Autodesk Inventor part; units mm, degrees
ref_plane "YZ Plane" through (0, 0, 0) normal (1, 0, 0) x (0, 1, 0)
ref_plane "XZ Plane" through (0, 0, 0) normal (0, 1, 0) x (-1, 0, 0)
ref_plane "XY Plane" through (0, 0, 0) normal (0, 0, 1) x (1, 0, 0)
sketch "Эскиз1" plane through (0, 0, 0) normal (0, 0, 1) x (1, 0, 0)
  arc A0 (130.1731, 0.7623) -> (123.4106, 7.5248) centre (123.4106, 0.7623) ccw
  line L0 (-123.2839, 7.5248) -> (123.4106, 7.5248)
  arc A1 (-123.2839, 7.5248) -> (-130.0464, 0.7623) centre (-123.2839, 0.7623) ccw
  line L1 (-130.0464, -1.7127) -> (-130.0464, 0.7623)
  arc A2 (-130.0464, -1.7127) -> (-123.2839, -8.4752) centre (-123.2839, -1.7127) ccw
  line L2 (123.4106, -8.4752) -> (-123.2839, -8.4752)
  arc A3 (123.4106, -8.4752) -> (130.1731, -1.7127) centre (123.4106, -1.7127) ccw
  line L3 (130.1731, 0.7623) -> (130.1731, -1.7127)
  circle A4 centre (122.1731, -0.4752) radius 1.85
  circle A5 centre (-124.1763, -0.4762) radius 1.65
  circle A6 centre (-106.5766, -0.4757) radius 2.65
  circle A7 centre (-92.1769, -0.4756) radius 1.65
  line L4 (-73.2645, 4.044) -> (-78.5234, -4.9714)
  arc A8 (-71.5369, 4.044) -> (-73.2645, 4.044) centre (-72.4007, 3.5401) ccw
  line L5 (-66.2779, -4.9714) -> (-71.5369, 4.044)
  arc A9 (-67.1417, -6.4752) -> (-66.2779, -4.9714) centre (-67.1417, -5.4752) ccw
  line L6 (-77.6596, -6.4752) -> (-67.1417, -6.4752)
  arc A10 (-78.5234, -4.9714) -> (-77.6596, -6.4752) centre (-77.6596, -5.4752) ccw
  line L7 (-57.8267, 5.5248) -> (-68.3446, 5.5248)
  arc A11 (-56.9629, 4.0209) -> (-57.8267, 5.5248) centre (-57.8267, 4.5248) ccw
  line L8 (-62.2219, -4.9945) -> (-56.9629, 4.0209)
  arc A12 (-63.9495, -4.9945) -> (-62.2219, -4.9945) centre (-63.0857, -4.4906) ccw
  line L9 (-69.2084, 4.0209) -> (-63.9495, -4.9945)
  arc A13 (-68.3446, 5.5248) -> (-69.2084, 4.0209) centre (-68.3446, 4.5248) ccw
  line L10 (-54.634, 4.044) -> (-59.893, -4.9714)
  arc A14 (-52.9065, 4.044) -> (-54.634, 4.044) centre (-53.7703, 3.5401) ccw
  line L11 (-47.6475, -4.9714) -> (-52.9065, 4.044)
  arc A15 (-48.5113, -6.4752) -> (-47.6475, -4.9714) centre (-48.5113, -5.4752) ccw
  line L12 (-59.0292, -6.4752) -> (-48.5113, -6.4752)
  arc A16 (-59.893, -4.9714) -> (-59.0292, -6.4752) centre (-59.0292, -5.4752) ccw
  line L13 (-39.1963, 5.5248) -> (-49.7142, 5.5248)
  arc A17 (-38.3325, 4.0209) -> (-39.1963, 5.5248) centre (-39.1963, 4.5248) ccw
  line L14 (-43.5915, -4.9945) -> (-38.3325, 4.0209)
  arc A18 (-45.319, -4.9945) -> (-43.5915, -4.9945) centre (-44.4553, -4.4906) ccw
  line L15 (-50.578, 4.0209) -> (-45.319, -4.9945)
  arc A19 (-49.7142, 5.5248) -> (-50.578, 4.0209) centre (-49.7142, 4.5248) ccw
  line L16 (-36.0036, 4.044) -> (-41.2626, -4.9714)
  arc A20 (-34.2761, 4.044) -> (-36.0036, 4.044) centre (-35.1399, 3.5401) ccw
  line L17 (-29.0171, -4.9714) -> (-34.2761, 4.044)
  arc A21 (-29.8809, -6.4752) -> (-29.0171, -4.9714) centre (-29.8809, -5.4752) ccw
  line L18 (-40.3988, -6.4752) -> (-29.8809, -6.4752)
  arc A22 (-41.2626, -4.9714) -> (-40.3988, -6.4752) centre (-40.3988, -5.4752) ccw
  line L19 (-20.5659, 5.5248) -> (-31.0838, 5.5248)
  arc A23 (-19.7021, 4.0209) -> (-20.5659, 5.5248) centre (-20.5659, 4.5248) ccw
  line L20 (-24.9611, -4.9945) -> (-19.7021, 4.0209)
  arc A24 (-26.6886, -4.9945) -> (-24.9611, -4.9945) centre (-25.8249, -4.4906) ccw
  line L21 (-31.9476, 4.0209) -> (-26.6886, -4.9945)
  arc A25 (-31.0838, 5.5248) -> (-31.9476, 4.0209) centre (-31.0838, 4.5248) ccw
  line L22 (-17.3732, 4.044) -> (-22.6322, -4.9714)
  arc A26 (-15.6457, 4.044) -> (-17.3732, 4.044) centre (-16.5095, 3.5401) ccw
  line L23 (-10.3867, -4.9714) -> (-15.6457, 4.044)
  arc A27 (-11.2505, -6.4752) -> (-10.3867, -4.9714) centre (-11.2505, -5.4752) ccw
  line L24 (-21.7684, -6.4752) -> (-11.2505, -6.4752)
  arc A28 (-22.6322, -4.9714) -> (-21.7684, -6.4752) centre (-21.7684, -5.4752) ccw
  line L25 (-1.9355, 5.5248) -> (-12.4534, 5.5248)
  arc A29 (-1.0717, 4.0209) -> (-1.9355, 5.5248) centre (-1.9355, 4.5248) ccw
  line L26 (-6.3307, -4.9945) -> (-1.0717, 4.0209)
  arc A30 (-8.0582, -4.9945) -> (-6.3307, -4.9945) centre (-7.1945, -4.4906) ccw
  line L27 (-13.3172, 4.0209) -> (-8.0582, -4.9945)
  arc A31 (-12.4534, 5.5248) -> (-13.3172, 4.0209) centre (-12.4534, 4.5248) ccw
  line L28 (113.0396, 4.044) -> (107.7807, -4.9714)
  arc A32 (114.7672, 4.044) -> (113.0396, 4.044) centre (113.9034, 3.5401) ccw
  line L29 (120.0261, -4.9714) -> (114.7672, 4.044)
  arc A33 (119.1624, -6.4752) -> (120.0261, -4.9714) centre (119.1624, -5.4752) ccw
  line L30 (108.6444, -6.4752) -> (119.1624, -6.4752)
  arc A34 (107.7807, -4.9714) -> (108.6444, -6.4752) centre (108.6444, -5.4752) ccw
  line L31 (1.2572, 4.044) -> (-4.0018, -4.9714)
  arc A35 (2.9847, 4.044) -> (1.2572, 4.044) centre (2.121, 3.5401) ccw
  line L32 (8.2437, -4.9714) -> (2.9847, 4.044)
  arc A36 (7.3799, -6.4752) -> (8.2437, -4.9714) centre (7.3799, -5.4752) ccw
  line L33 (-3.138, -6.4752) -> (7.3799, -6.4752)
  arc A37 (-4.0018, -4.9714) -> (-3.138, -6.4752) centre (-3.138, -5.4752) ccw
  line L34 (16.6949, 5.5248) -> (6.177, 5.5248)
  arc A38 (17.5587, 4.0209) -> (16.6949, 5.5248) centre (16.6949, 4.5248) ccw
  line L35 (12.2997, -4.9945) -> (17.5587, 4.0209)
  arc A39 (10.5722, -4.9945) -> (12.2997, -4.9945) centre (11.436, -4.4906) ccw
  line L36 (5.3132, 4.0209) -> (10.5722, -4.9945)
  arc A40 (6.177, 5.5248) -> (5.3132, 4.0209) centre (6.177, 4.5248) ccw
  line L37 (98.4652, 4.0209) -> (103.7242, -4.9945)
  arc A41 (99.329, 5.5248) -> (98.4652, 4.0209) centre (99.329, 4.5248) ccw
  line L38 (109.847, 5.5248) -> (99.329, 5.5248)
  arc A42 (110.7107, 4.0209) -> (109.847, 5.5248) centre (109.847, 4.5248) ccw
  line L39 (105.4518, -4.9945) -> (110.7107, 4.0209)
  arc A43 (103.7242, -4.9945) -> (105.4518, -4.9945) centre (104.588, -4.4906) ccw
  line L40 (94.4092, 4.044) -> (89.1502, -4.9714)
  arc A44 (96.1368, 4.044) -> (94.4092, 4.044) centre (95.273, 3.5401) ccw
  line L41 (101.3957, -4.9714) -> (96.1368, 4.044)
  arc A45 (100.532, -6.4752) -> (101.3957, -4.9714) centre (100.532, -5.4752) ccw
  line L42 (90.014, -6.4752) -> (100.532, -6.4752)
  arc A46 (89.1502, -4.9714) -> (90.014, -6.4752) centre (90.014, -5.4752) ccw
  line L43 (19.8876, 4.044) -> (14.6286, -4.9714)
  arc A47 (21.6151, 4.044) -> (19.8876, 4.044) centre (20.7514, 3.5401) ccw
  line L44 (26.8741, -4.9714) -> (21.6151, 4.044)
  arc A48 (26.0103, -6.4752) -> (26.8741, -4.9714) centre (26.0103, -5.4752) ccw
  line L45 (15.4924, -6.4752) -> (26.0103, -6.4752)
  arc A49 (14.6286, -4.9714) -> (15.4924, -6.4752) centre (15.4924, -5.4752) ccw
  line L46 (35.3253, 5.5248) -> (24.8074, 5.5248)
  arc A50 (36.1891, 4.0209) -> (35.3253, 5.5248) centre (35.3253, 4.5248) ccw
  line L47 (30.9301, -4.9945) -> (36.1891, 4.0209)
  arc A51 (29.2026, -4.9945) -> (30.9301, -4.9945) centre (30.0664, -4.4906) ccw
  line L48 (23.9436, 4.0209) -> (29.2026, -4.9945)
  arc A52 (24.8074, 5.5248) -> (23.9436, 4.0209) centre (24.8074, 4.5248) ccw
  line L49 (79.8348, 4.0209) -> (85.0938, -4.9945)
  arc A53 (80.6986, 5.5248) -> (79.8348, 4.0209) centre (80.6986, 4.5248) ccw
  line L50 (91.2165, 5.5248) -> (80.6986, 5.5248)
  arc A54 (92.0803, 4.0209) -> (91.2165, 5.5248) centre (91.2165, 4.5248) ccw
  line L51 (86.8214, -4.9945) -> (92.0803, 4.0209)
  arc A55 (85.0938, -4.9945) -> (86.8214, -4.9945) centre (85.9576, -4.4906) ccw
  line L52 (75.7788, 4.044) -> (70.5198, -4.9714)
  arc A56 (77.5064, 4.044) -> (75.7788, 4.044) centre (76.6426, 3.5401) ccw
  line L53 (82.7653, -4.9714) -> (77.5064, 4.044)
  arc A57 (81.9015, -6.4752) -> (82.7653, -4.9714) centre (81.9015, -5.4752) ccw
  line L54 (71.3836, -6.4752) -> (81.9015, -6.4752)
  arc A58 (70.5198, -4.9714) -> (71.3836, -6.4752) centre (71.3836, -5.4752) ccw
  line L55 (38.518, 4.044) -> (33.259, -4.9714)
  arc A59 (40.2455, 4.044) -> (38.518, 4.044) centre (39.3818, 3.5401) ccw
  line L56 (45.5045, -4.9714) -> (40.2455, 4.044)
  arc A60 (44.6407, -6.4752) -> (45.5045, -4.9714) centre (44.6407, -5.4752) ccw
  line L57 (34.1228, -6.4752) -> (44.6407, -6.4752)
  arc A61 (33.259, -4.9714) -> (34.1228, -6.4752) centre (34.1228, -5.4752) ccw
  line L58 (53.9557, 5.5248) -> (43.4378, 5.5248)
  arc A62 (54.8195, 4.0209) -> (53.9557, 5.5248) centre (53.9557, 4.5248) ccw
  line L59 (49.5605, -4.9945) -> (54.8195, 4.0209)
  arc A63 (47.833, -4.9945) -> (49.5605, -4.9945) centre (48.6968, -4.4906) ccw
  line L60 (42.574, 4.0209) -> (47.833, -4.9945)
  arc A64 (43.4378, 5.5248) -> (42.574, 4.0209) centre (43.4378, 4.5248) ccw
  line L61 (61.2044, 4.0209) -> (66.4634, -4.9945)
  arc A65 (62.0682, 5.5248) -> (61.2044, 4.0209) centre (62.0682, 4.5248) ccw
  line L62 (72.5861, 5.5248) -> (62.0682, 5.5248)
  arc A66 (73.4499, 4.0209) -> (72.5861, 5.5248) centre (72.5861, 4.5248) ccw
  line L63 (68.191, -4.9945) -> (73.4499, 4.0209)
  arc A67 (66.4634, -4.9945) -> (68.191, -4.9945) centre (67.3272, -4.4906) ccw
  line L64 (57.1484, 4.044) -> (51.8894, -4.9714)
  arc A68 (58.876, 4.044) -> (57.1484, 4.044) centre (58.0122, 3.5401) ccw
  line L65 (64.1349, -4.9714) -> (58.876, 4.044)
  arc A69 (63.2711, -6.4752) -> (64.1349, -4.9714) centre (63.2711, -5.4752) ccw
  line L66 (52.7532, -6.4752) -> (63.2711, -6.4752)
  arc A70 (51.8894, -4.9714) -> (52.7532, -6.4752) centre (52.7532, -5.4752) ccw
  line L67 (122.1731, -0.4752) -> (92.1731, -0.4752)
  circle A71 centre (92.1731, -0.4752) radius 1.85
  arc A72 (100.1731, 0.7623) -> (93.4106, 7.5248) centre (93.4106, 0.7623) ccw
  arc A73 (93.4106, -8.4752) -> (100.1731, -1.7127) centre (93.4106, -1.7127) ccw
  line L68 (100.1731, 0.7623) -> (100.1731, -1.7127)
  point P0 (0, 0)
  point P1 (6.1731, -0.4752)
  point P2 (93.4106, -8.4752)
  dimension "d0" = 30
extrude "Выдавливание1" add sketch "Эскиз1" along normal blind 3.2 contours A72 A41 L37 L68 L67 L41 A44 L40 A71 A46 L42 A73 L2 A2 L1 A1 L0 | A72 L37 A41 | L42 A46 L40 A71 L67 L41 A73 | L41 L67 L68 A73 | L67 A71 L40 A44 L41 | A8 L5 A9 L6 A10 L4 | A11 L8 A12 L9 A13 L7 | A14 L11 A15 L12 A16 L10 | A17 L14 A18 L15 A19 L13 | A20 L17 A21 L18 A22 L16 | A23 L20 A24 L21 A25 L19 | A26 L23 A27 L24 A28 L22 | A29 L26 A30 L27 A31 L25 | A35 L32 A36 L33 A37 L31 | A38 L35 A39 L36 A40 L34 | A47 L44 A48 L45 A49 L43 | A50 L47 A51 L48 A52 L46 | A53 L50 A54 L51 A55 L49 | A56 L53 A57 L54 A58 L52 | A59 L56 A60 L57 A61 L55 | A62 L59 A63 L60 A64 L58 | A65 L62 A66 L63 A67 L61 | A68 L65 A69 L66 A70 L64
sketch "Эскиз2" plane through (0, 0, 3.2) normal (0, 0, 1) x (1, 0, 0)
  line L0 (100.1731, -1.7127) -> (100.1731, 0.7623)
  arc A0 (100.1731, 0.7623) -> (93.4106, 7.5248) centre (93.4106, 0.7623) ccw
  line L1 (93.4106, 7.5248) -> (-123.2839, 7.5248)
  arc A1 (-123.2839, 7.5248) -> (-130.0464, 0.7623) centre (-123.2839, 0.7623) ccw
  line L2 (-130.0464, 0.7623) -> (-130.0464, -1.7127)
  arc A2 (-130.0464, -1.7127) -> (-123.2839, -8.4752) centre (-123.2839, -1.7127) ccw
  line L3 (-123.2839, -8.4752) -> (93.4106, -8.4752)
  arc A3 (93.4106, -8.4752) -> (100.1731, -1.7127) centre (93.4106, -1.7127) ccw
  circle A4 centre (92.1731, -0.4752) radius 1.85
  circle A5 centre (-106.5766, -0.4757) radius 2.65
  circle A6 centre (-92.1769, -0.4756) radius 1.65
  circle A7 centre (-124.1763, -0.4762) radius 1.65
  line L4 (-128.0657, -6.4946) -> (127, -6.4946)
  line L5 (-124.1763, -0.4762) -> (-92.1769, -0.4756)
  line L6 (-130.0464, 5.5419) -> (126.9998, 5.5522)
  point P0 (0, 0)
  point P1 (-128.0659, 5.542)
  point P2 (98.1924, -6.4946)
  point P3 (-128.0678, 5.542)
  point P4 (98.1854, 5.551)
extrude "Выдавливание2" cut sketch "Эскиз2" against normal blind 3.2 contours A3 L3 A2 L4 | L6 A1 L1 A0
fillet "Сопряжение1" radius 2 4 edges at (-128.0657, -6.4946, 1.6) (-128.0678, 5.542, 1.6) (98.1854, 5.551, 1.6) (98.1924, -6.4946, 1.6)
properties part number "ДЛЯ ПОДВЕСА"
Geometry check sheet. Reference: the model listing, model coordinates, mm. Give positions to 0.01 mm unless a question says otherwise; leave off trailing zeros.
1) Release check for a two-part mould opening along X. For faces 1 (the cylindrical face through (93.882, 0.233, 1.578)), 2 (the flat face through (-17, 0, 0)) record: pulls with the +X half, pulls with the -X half, needs draft (parallel to the pull), parting line crosses it, or undercut.
2) Material ranges on L1, parallel to X at y = -0.25, z = 0.2; L2, parallel to Y at x = -47, z = 0.75; L3, parallel to X at y = 1, z = 2.1, recorded low to high.
3) Gauge pin test, flat end, axial feed: pin 1 (1 mm diameter, centred on x = 1.5, z = 2, fed in from +Y). Record the tip position at first contact, or that the pin passes through.
4) Section check A-A, the plane z = 0.7. State how many separate pieces and enclosed holes the cut face has, and give its area (3 significant figures).
Computed:
1. face 1: undercut
1. face 2: needs draft
2. L1: x = -130.05 to -125.81, -122.54 to -109.22, -103.94 to -93.81, -90.54 to 90.34, 94.01 to 100.17
2. L2: y = -6.49 to 5.55
2. L3: x = -130.04 to -124.91, -123.44 to -108.78, -104.38 to -92.92, -91.44 to 91.06, 93.29 to 100.17
3. pin 1: stops at y = 5.55
4. separate pieces: 1
4. enclosed holes: 4
4. area: 2,710 mm2
